```python
from build123d import *

# Parameters (mm, degrees)
F0_W     = 50
F0_H     = 100
F0_R     = 10
F1_DEPTH = 30
F2_W     = 50
F2_H     = 10
F3_DEPTH = 5
F5_DEPTH = 50
F6_R     = 10
F7_DEPTH = 15


with BuildPart() as f1:
    # F0 (on Top) → F1 (new body)
    with BuildSketch(Plane.XY):
        Rectangle(F0_W, F0_H)
        Circle(F0_R, mode=Mode.SUBTRACT)
    extrude(amount=F1_DEPTH)

    # F2 (on face) → F3 (cut)
    with BuildSketch(Plane.XY.offset(30)):
        with BuildLine():
            Line((7.806247498, -6.25), (25, -6.25))
            Line((25, -6.25), (25, 6.25))
            Line((25, 6.25), (7.806247498, 6.25))
            ThreePointArc((7.806247498, 6.25), (9.4356365705, 3.3119122135), (10, 0))
            ThreePointArc((10, 0), (9.4356365705, -3.3119122135), (7.806247498, -6.25))
        make_face()
        with Locations((0, -30)):
            Rectangle(F2_W, F2_H)
        with BuildLine():
            Line((-25, 6.25), (-25, -6.25))
            Line((-25, -6.25), (-7.806247498, -6.25))
            ThreePointArc((-7.806247498, -6.25), (-10, 0), (-7.806247498, 6.25))
            Line((-7.806247498, 6.25), (-25, 6.25))
        make_face()
    extrude(amount=-F3_DEPTH, mode=Mode.SUBTRACT)

    # F4 (on face) → F5 (cut, through all)
    with BuildSketch(Plane(origin=(-25, 0, 0), x_dir=(0, -1, 0), z_dir=(-1, 0, 0))):
        Polygon((-22.5, 30), (-37.5, 30), (-43.2735026919, 20), (-16.7264973081, 20), align=None)
    extrude(amount=-F5_DEPTH, mode=Mode.SUBTRACT)

    # F6 (on face) → F7 (join)
    with BuildSketch(Plane(origin=(0, 50, 0), x_dir=(-1, 0, 0), z_dir=(0, 1, 0))):
        with Locations((0, 15)):
            Circle(F6_R)
    extrude(amount=F7_DEPTH)


solid = f1.part
```
Source: CAD feature listing. Evaluate the final solid. Frame: model axes, mm. A direction names the side the tool comes from. Give positions to 0.01 mm unless a question says otherwise; leave off trailing zeros. Loops run counter-clockwise (first coordinate to the right, second up) from the corner with the lowest first, then second, coordinate; pieces in that order, holes last. Notation, with made-up numbers: (11, 14.25) -> (43, 14.25) arc R27 cw to (43, 34.25) -> close; hole circle Ø10 at (-28, -5.5). An arc over 180 degrees is marked (long way). Use a Markdown table: item, result. Add a question column.
(1) Section query C-C (z = 15). Output: boundary loops of the cut face in (x, y), then the cut area to 3 significant figures.
(2) Access query for faces 1 (the face through (1.302, 57.395, 24.915)), 2 (the face through (-0.35, 40.346, 25.07)), 3 (the face through (0, -35, 28)). Directions: +Z, -Z, +X, -X, +Y, -Y. A direction counts if a zero-diameter tool reaches every point of the face in a straight line with its end or side. Return the directions, or none.
(3) Section query B-B (y = 0). Output: boundary loops of the cut face in (x, z), then the cut area to 3 significant figures.
(4) First-contact query: pin 1 Ø18 at (x, y) = (0, 0) entering from +Z; pin 2 Ø4 at (x, z) = (-10, 27) entering from +Y; pin 3 Ø4 at (x, y) = (12, -1.5) entering from +Z. Flat tips, straight axial feed; report the tip coordinate or a pass-through.
(5) Pull-direction query (Y, two-part tool) for faces 4 (the face through (-25, -1, 15)), 5 (the face through (16, 0, 25)), 6 (the face through (-0.3, 50, 4.8)); classes: +Y half, -Y half, draft (parallel to the pull), parting line (faces both ways), or undercut.
(6) Ray query, line 1 (Y direction, x = 0, z = 15.25); line 2 (X direction, y = 0, z = 19.75); line 3 (Y direction, x = 0, z = 22.25). Return the intervals inside material, ascending.
(7) Section query D-D (z = 22.75). Output: boundary loops of the cut face in (x, y), then the cut area to 3 significant figures.
(8) Section query A-A (x = 0). Output: boundary loops of the cut face in (y, z).
Checked values:
| question | item | result |
|---|---|---|
| 1 | outline | (-25, -50) -> (25, -50) -> (25, 50) -> (10, 50) -> (10, 65) -> (-10, 65) -> (-10, 50) -> (-25, 50) -> close; hole circle Ø20 at (0, 0) |
| 1 | area | 4,990 mm^2 |
| 2 | face 1 | +Y |
| 2 | face 2 | +X, -X |
| 2 | face 3 | +Z, +X, -X |
| 3 | outline | (-25, 0) -> (-10, 0) -> (-10, 25) -> (-25, 25) -> close; (10, 0) -> (25, 0) -> (25, 25) -> (10, 25) -> close |
| 3 | area | 750 mm^2 |
| 4 | pin 1 | through |
| 4 | pin 2 | y = 50 |
| 4 | pin 3 | z = 25 |
| 5 | face 4 | draft |
| 5 | face 5 | undercut |
| 5 | face 6 | +Y half |
| 6 | line 1 | -50 to -10, 10 to 65 |
| 6 | line 2 | -25 to -10, 10 to 25 |
| 6 | line 3 | -50 to -10, 10 to 18.03, 41.97 to 65 |
| 7 | outline | (-25, -50) -> (25, -50) -> (25, 18.31) -> (-25, 18.31) -> close; (-25, 41.69) -> (25, 41.69) -> (25, 50) -> (6.32, 50) -> (6.32, 65) -> (-6.32, 65) -> (-6.32, 50) -> (-25, 50) -> close; hole circle Ø20 at (0, 0) |
| 7 | area | 3,710 mm^2 |
| 8 | outline | (-50, 0) -> (-10, 0) -> (-10, 30) -> (-25, 30) -> (-25, 25) -> (-35, 25) -> (-35, 30) -> (-50, 30) -> close; (10, 0) -> (50, 0) -> (50, 5) -> (65, 5) -> (65, 25) -> (50, 25) -> (50, 30) -> (37.5, 30) -> (43.27, 20) -> (16.73, 20) -> (22.5, 30) -> (10, 30) -> close |
